Design review of the part built by this model. Coordinates are the model's own, in mm. Face numbers are marked on the shaded views. A direction names the side the tool comes from. Give positions to 0.01 mm unless a question says otherwise; leave off trailing zeros. Write each loop counter-clockwise with the first axis right and the second up, starting at its lowest first coordinate (ties: lowest second). Pieces come first, ordered by that corner, then holes. Notation, with made-up numbers: M 82.5,32 L 93.5,32 A11 cw 93.5,51 Z; hole C 59.5,54 d9. An arc over 180 degrees is marked long. Answer in a Markdown table with one row per item.
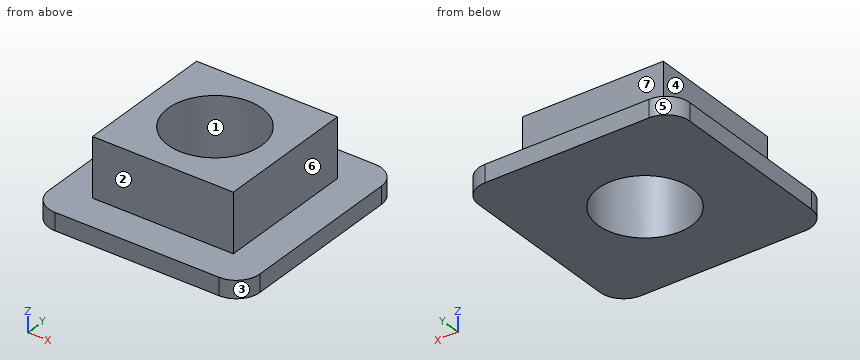
```python
from build123d import *

# Parameters (mm, degrees)
BOSS_EXTRUDE1_DEPTH = 1.5
SKETCH2_W           = 12
SKETCH2_H           = 12
BOSS_EXTRUDE2_DEPTH = 5
SKETCH3_R           = 4
CUT_EXTRUDE1_DEPTH  = 7.5


with BuildPart() as part:
    # Sketch1 → Boss-Extrude1 (new body)
    with BuildSketch(Plane.XY):
        with BuildLine():
            Line((2, 0), (16, 0))
            ThreePointArc((16, 0), (17.414213562, 0.585786438), (18, 2))
            Line((18, 2), (18, 16))
            ThreePointArc((18, 16), (17.414213562, 17.414213562), (16, 18))
            Line((16, 18), (2, 18))
            ThreePointArc((2, 18), (0.585786438, 17.414213562), (0, 16))
            Line((0, 16), (0, 2))
            ThreePointArc((0, 2), (0.585786438, 0.585786438), (2, 0))
        make_face()
    extrude(amount=BOSS_EXTRUDE1_DEPTH)

    # Sketch2 → Boss-Extrude2 (add)
    with BuildSketch(Plane.XY.offset(1.5)):
        with Locations((9, 9)):
            Rectangle(SKETCH2_W, SKETCH2_H)
    extrude(amount=BOSS_EXTRUDE2_DEPTH)

    # Sketch3 → Cut-Extrude1 (cut, through all)
    with BuildSketch(Plane.XY.offset(6.5)):
        with Locations((9, 9)):
            Circle(SKETCH3_R)
    extrude(amount=-CUT_EXTRUDE1_DEPTH, mode=Mode.SUBTRACT)


solid = part.part
```
1) The part is to be moulded in two halves that separate along X. For the marked faces 1, 2, 3 and 4, say which applies: released by +X, released by -X, zero draft, split by the parting line, or undercut.
Geometry says:
| item | result |
|---|---|
| face 1 | undercut |
| face 2 | zero draft |
| face 3 | released by +X |
| face 4 | released by -X |
2) Add section A-A (y = 9). Write out the cut boundary in (x, z), and give its area (3 significant figures).
Geometry says:
| item | result |
|---|---|
| outline | M 0,0 L 5,0 L 5,6.5 L 3,6.5 L 3,1.5 L 0,1.5 Z; M 13,0 L 18,0 L 18,1.5 L 15,1.5 L 15,6.5 L 13,6.5 Z |
| area | 35.0 mm^2 |
3) To check wall thickness, follow probe 1 along Y at (x, z) = (9, 3); probe 2 along Z at (x, y) = (2.25, 3.5); probe 3 along X at (y, z) = (6.5, 2). State the ranges of each line that lie inside material, in increasing order. Write a range as [from, to].
Geometry says:
| item | result |
|---|---|
| probe 1 | [3, 5], [13, 15] |
| probe 2 | [0, 1.5] |
| probe 3 | [3, 5.88], [12.12, 15] |
4) Add section B-B (z = 4). Write out the cut boundary in (x, y), and give its area (3 significant figures).
Geometry says:
| item | result |
|---|---|
| outline | M 3,3 L 15,3 L 15,15 L 3,15 Z; hole C 9,9 d8 |
| area | 93.7 mm^2 |
5) For the marked faces 5, 6 and 7, list the 3-axis set-ups (+Z, -Z, +X, -X, +Y, -Y) from which the entire face can be reached by the end or side of a thin tool; tool diameter is ignored.
Geometry says:
| item | result |
|---|---|
| face 5 | +Z, -Z, -X, +Y |
| face 6 | +Z, +X, +Y, -Y |
| face 7 | +Z, +X, -X, +Y |
6) Add section D-D (y = 13.25). Write out the cut boundary in (x, z), and give its area (3 significant figures).
Geometry says:
| item | result |
|---|---|
| outline | M 0,0 L 18,0 L 18,1.5 L 15,1.5 L 15,6.5 L 3,6.5 L 3,1.5 L 0,1.5 Z |
| area | 87.0 mm^2 |
7) Insertion check: P1, Ø1.5, axis at y = 7.5, z = 3.5, coming from the +X side. The pin has a flat end and moves straight along its axis. Give the tip position at first contact, or say it passes through.
Geometry says:
| item | result |
|---|---|
| P1 | x = 15 |
